Geometry: see drawing. Coordinates: mm, zero at the bounding-box minimum. A direction names the side the tool comes from. Coordinates: 2 decimals unless noted, no trailing zeros. Write each loop counter-clockwise with the first axis right and the second up, starting at its lowest first coordinate (ties: lowest second). Pieces come first, ordered by that corner, then holes. Notation, with made-up numbers: M 26,-28.5 L 58,-28.5 A6 cw 58,-23.5 Z; hole C 19.25,59 d4. An arc over 180 degrees is marked long. One line per item, written item: value. Start each with the question number.
Item 1: Cut plane B-B, the plane y = 33. Output: boundary loops of the cut face in (x, z), then the cut area to 3 significant figures.
Item 2: Cut plane D-D, the plane y = 38. Output: boundary loops of the cut face in (x, z) (1 decimal), then the cut area to 3 significant figures.
Item 3: Cut plane C-C, the plane x = 18.5. Output: boundary loops of the cut face in (y, z).
Item 4: Pin query (flat end, axial travel): P1, Ø5, axis at y = 13, z = 8, coming from the -X side; P2, Ø1.5, axis at x = 63.5, z = 13.5, coming from the +Y side; P3, Ø10, axis at x = 61, y = 17.5, coming from the +Z side; P4, Ø6.5, axis at x = 24, z = 39.5, coming from the +Y side. Return the tip coordinate at first contact, or that it passes through.
Item 5: Mould query, pull axis Y, two halves, no side actions, for the marked faces 6, 7, 8 and 9. Classes: released by +Y, released by -Y, zero draft, split by the parting line, or undercut.
Item 6: Set-up query: the marked faces 1, 2, 3, 4 and 5. Return all of +Z, -Z, +X, -X, +Y, -Y with unobstructed straight access to the full face (end or side cutting, diameter ignored); none if empty.
Item 7: Ray query, L1, parallel to Z at x = 9, y = 25; L2, parallel to X at y = 33, z = 46 (1 decimal); L3, parallel to Y at x = 17.5, z = 12 (1 decimal). Return the intervals inside material, ascending. Write a range as from..to.
Item 8: Cut plane A-A, the plane z = 44.5. Output: boundary loops of the cut face in (x, y).
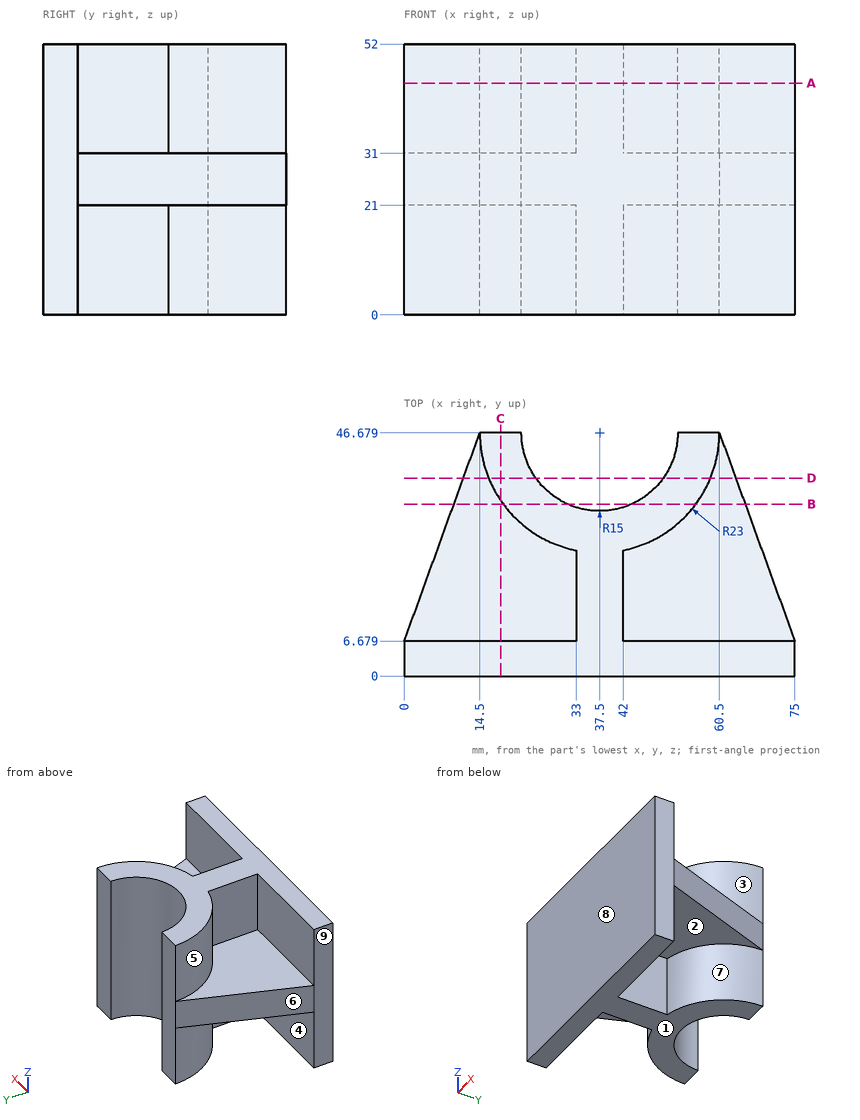
From the geometry:
1. outline: M 9.54,21 L 19.01,21 L 19.01,0 L 31.34,0 L 31.34,52 L 19.01,52 L 19.01,31 L 9.54,31 Z; M 43.66,0 L 55.99,0 L 55.99,21 L 65.46,21 L 65.46,31 L 55.99,31 L 55.99,52 L 43.66,52 Z
1. area: 1,470 mm²
2. outline: M 11.4,21 L 16.2,21 L 16.2,0 L 25.3,0 L 25.3,52 L 16.2,52 L 16.2,31 L 11.4,31 Z; M 49.7,0 L 58.8,0 L 58.8,21 L 63.6,21 L 63.6,31 L 58.8,31 L 58.8,52 L 49.7,52 Z
2. area: 1,040 mm²
3. outline: M 0,0 L 6.68,0 L 6.68,21 L 33.72,21 L 33.72,0 L 46.68,0 L 46.68,52 L 33.72,52 L 33.72,31 L 6.68,31 L 6.68,52 L 0,52 Z
4. P1: stops at x = 33
4. P2: stops at y = 6.68
4. P3: stops at z = 31
4. P4: stops at y = 46.68
5. face 6: released by +Y
5. face 7: undercut
5. face 8: released by -Y
5. face 9: zero draft
6. face 1: -Z, +X, -X, +Y, -Y
6. face 2: -Z, +X
6. face 3: +Z, +X
6. face 4: -Z, -X
6. face 5: +Z, -X
7. L1: z = 21..31
7. L2: x = 19..31.3, 43.7..56
7. L3: y = 0..6.7, 35.3..46.7
8. outline: M 0,0 L 75,0 L 75,6.68 L 42,6.68 L 42,24.12 A23 ccw 60.5,46.68 L 52.5,46.68 A15 cw 22.5,46.68 L 14.5,46.68 A23 ccw 33,24.12 L 33,6.68 L 0,6.68 Z
